```python
from build123d import *

# Parameters (mm, degrees)
F0_W     = 103
F0_H     = 99
F3_DEPTH = 3
F1_W     = 79
F1_H     = 52
F4_DEPTH = 3.001
F2_W     = 12
F2_H     = 12
F5_DEPTH = 3.001
F6_R     = 1
F7_DEPTH = 3.001


with BuildPart() as f3:
    # F0 (on Top) → F3 (new body)
    with BuildSketch(Plane.XY):
        with Locations((1.623269, -13.150178)):
            Rectangle(F0_W, F0_H)
    extrude(amount=-F3_DEPTH)

    # F1 (on face) → F4 (cut, through all)
    with BuildSketch(Plane.XY):
        with Locations((2.123269, -1.650178)):
            Rectangle(F1_W, F1_H)
    extrude(amount=-F4_DEPTH, mode=Mode.SUBTRACT)

    # F2 (on Top) → F5 (cut, through all)
    with BuildSketch(Plane.XY):
        with Locations((26.123269, -43.650178)):
            Rectangle(F2_W, F2_H)
    extrude(amount=-F5_DEPTH, mode=Mode.SUBTRACT)

    # F6 (on face) → F7 (cut, through all)
    with BuildSketch(Plane.XY):
        with Locations((-42.876731, 29.349822)):
            Circle(F6_R)
        with Locations((-134.126731, 29.349822)):
            Circle(F6_R)
        with Locations((46.123269, 29.349822)):
            Circle(F6_R)
        with Locations((-42.876731, -55.650178)):
            Circle(F6_R)
        with Locations((46.123269, -55.650178)):
            Circle(F6_R)
    extrude(amount=-F7_DEPTH, mode=Mode.SUBTRACT)


solid = f3.part
```
Geometry check sheet. Reference: the model listing, model coordinates, mm. A direction names the side the tool comes from. Give positions to 0.01 mm unless a question says otherwise; leave off trailing zeros. Loops run counter-clockwise (first coordinate to the right, second up) from the corner with the lowest first, then second, coordinate; pieces in that order, holes last. Notation, with made-up numbers: M -39,46.25 L -12,46.25 A21 ccw -12,83.25 Z; hole C 2,16 d6. An arc over 180 degrees is marked long. Write item = value, one per line.
(1) Material ranges on line 1 (Y direction, x = 28, z = -1.45); line 2 (Y direction, x = 46, z = -2.4); line 3 (Y direction, x = -24, z = -0.8), recorded low to high. Write a range as [from, to].
Answer below:
line_1 = [-62.65, -49.65], [-37.65, -27.65], [24.35, 36.35]
line_2 = [-62.65, -56.64], [-54.66, 28.36], [30.34, 36.35]
line_3 = [-62.65, -27.65], [24.35, 36.35]
(2) Sectioned sample at D-D, the plane z = -1.45. Record the cut outline in (x, y).
Answer below:
outline = M -49.88,-62.65 L 53.12,-62.65 L 53.12,36.35 L -49.88,36.35 Z; hole C -42.88,-55.65 d2; hole C -42.88,29.35 d2; hole M -37.38,-27.65 L 41.62,-27.65 L 41.62,24.35 L -37.38,24.35 Z; hole M 20.12,-49.65 L 32.12,-49.65 L 32.12,-37.65 L 20.12,-37.65 Z; hole C 46.12,-55.65 d2; hole C 46.12,29.35 d2
(3) Tool access check on faces 5 (the face through (26, -49.65, -1)), 6 (the face through (53.123, -14, -1)). Record the directions out of +Z, -Z, +X, -X, +Y, -Y that give a thin tool (end or side, any length) a straight path to the whole face; none if there is none.
Answer below:
face_5 = +Z, -Z
face_6 = +Z, -Z, +X, +Y, -Y
(4) Sectioned sample at B-B, the plane y = -4.5. Record the cut outline in (x, z), plus the area to 3 significant figures.
Answer below:
outline = M -49.88,-3 L -37.38,-3 L -37.38,0 L -49.88,0 Z; M 41.62,-3 L 53.12,-3 L 53.12,0 L 41.62,0 Z
area = 72.0 mm2
(5) Gauge pin test, flat ends, axial feed: pin 1 Ø2.5 at (x, y) = (-42.88, -55.65) entering from -Z; pin 2 Ø1.8 at (x, y) = (46.12, 29.35) entering from +Z. Record the tip position at first contact, or that the pin passes through.
Answer below:
pin_1 = -3
pin_2 = through
(6) Sectioned sample at C-C, the plane x = -19. Record the cut outline in (y, z).
Answer below:
outline = M -62.65,-3 L -27.65,-3 L -27.65,0 L -62.65,0 Z; M 24.35,-3 L 36.35,-3 L 36.35,0 L 24.35,0 Z
(7) Release check for a two-part mould opening along Y. For faces 1 (the face through (1, -62.65, -1)), 2 (the face through (-49.877, -14, -1)), 3 (the face through (-37.377, -2, -1)), 4 (the face through (32.123, -44, -1)) record: released by +Y, released by -Y, zero draft, split by the parting line, or undercut.
Answer below:
face_1 = released by -Y
face_2 = zero draft
face_3 = undercut
face_4 = undercut
(8) Sectioned sample at A-A, the plane x = 26. Record the cut outline in (y, z).
Answer below:
outline = M -62.65,-3 L -49.65,-3 L -49.65,0 L -62.65,0 Z; M -37.65,-3 L -27.65,-3 L -27.65,0 L -37.65,0 Z; M 24.35,-3 L 36.35,-3 L 36.35,0 L 24.35,0 Z
